Input: part model. Units: mm. Frame: model coordinates. A direction names the side the tool comes from. Round coordinates to 2 decimals unless told otherwise and drop trailing zeros. Loops run counter-clockwise (first coordinate to the right, second up) from the corner with the lowest first, then second, coordinate; pieces in that order, holes last. Notation, with made-up numbers: M 49.25,-27.75 L 83.25,-27.75 A21 cw 83.25,-19.75 Z; hole C 29.25,53 d4. An arc over 180 degrees is marked long. Use one line per item in the form item = value. Start each with the question number.
Q1. Access query for faces 1 (the cylindrical face through (-46.122, -24.331, -26.533)), 2 (the cylindrical face through (55.506, 7.509, -23.846)), 3 (the flat face through (73.5, -8, -24)), 4 (the flat face through (-19, 22, 6)), 5 (the flat face through (-73.5, -15, -15)). Directions: +Z, -Z, +X, -X, +Y, -Y. A direction counts if a zero-diameter tool reaches every point of the face in a straight line with its end or side. Return the directions, or none.
Q2. First-contact query: P1, Ø24.5, axis at y = 6, z = -4, coming from the +X side; P2, Ø3.5, axis at x = -6, y = 22.5, coming from the -Z side; P3, Ø8, axis at x = -39.5, y = 9, coming from the +Z side; P4, Ø3.5, axis at x = 2.5, z = 2.5, coming from the -Y side. Flat tips, straight axial feed; report the tip coordinate or a pass-through.
Q3. Section query A-A, the plane z = 0. Output: boundary loops of the cut face in (x, y).
Q4. Section query C-C, the plane x = -5. Output: boundary loops of the cut face in (y, z), and give its area (3 significant figures).
Q5. Section query B-B, the plane y = 0. Output: boundary loops of the cut face in (x, z), and give its area (3 significant figures).
Q6. Mould query, pull axis Y, two halves, no side actions, for faces 6 (the cylindrical face through (27.65, 37.18, 4.88)), 7 (the flat face through (-19.5, -14, 34)), 8 (the cylindrical face through (-17.73, -20.983, 0.838)). Classes: pulls with the +Y half, pulls with the -Y half, needs draft (parallel to the pull), parting line crosses it, or undercut.
Q7. Section query D-D, the plane y = 32. Output: boundary loops of the cut face in (x, z), and give its area (3 significant figures).
Q8. Ray query, line 1 along Z through (x, y) = (51.5, 0); line 2 along Z through (x, y) = (14, 4). Return the intervals inside material, ascending.
```python
from build123d import *

# Parameters (mm, degrees)
SKETCH1_R           = 37.5
BOSS_EXTRUDE1_DEPTH = 73.5
SKETCH2_R           = 21
CUT_EXTRUDE1_DEPTH  = 157.273798188
SKETCH3_R           = 25
CUT_EXTRUDE2_DEPTH  = 36.5
SKETCH4_W           = 12
SKETCH4_H           = 20.96554604
CUT_EXTRUDE3_DEPTH  = 110.5
FILLET1_R           = 0.5
SKETCH5_W           = 54
SKETCH5_H           = 1.5


with BuildPart() as part:
    # Sketch1 → Boss-Extrude1 (new, symmetric)
    with BuildSketch(Plane(origin=(0, 0, 0), x_dir=(0, 0, -1), z_dir=(1, 0, 0))):
        Circle(SKETCH1_R)
    extrude(amount=BOSS_EXTRUDE1_DEPTH, both=True)

    # Sketch2 → Cut-Extrude1 (cut, through all)
    with BuildSketch(Plane(origin=(73.5, 0, 0), x_dir=(0, 0, -1), z_dir=(1, 0, 0))):
        Circle(SKETCH2_R)
    extrude(amount=-CUT_EXTRUDE1_DEPTH, mode=Mode.SUBTRACT)

    # Sketch3 → Cut-Extrude2 (cut)
    with BuildSketch(Plane(origin=(73.5, 0, 0), x_dir=(0, 0, -1), z_dir=(1, 0, 0))):
        Circle(SKETCH3_R)
    extrude(amount=-CUT_EXTRUDE2_DEPTH, mode=Mode.SUBTRACT)

    # Sketch4 → Cut-Extrude3 (cut)
    with BuildSketch(Plane.ZY.offset(73.5)):
        with Locations((0, 13.81722698)):
            Rectangle(SKETCH4_W, SKETCH4_H)
    extrude(amount=-CUT_EXTRUDE3_DEPTH, mode=Mode.SUBTRACT)

    # Fillet1
    fillet1_edges = [part.edges().sort_by_distance(p)[0] for p in [
        (37, -21, 0),
    ]]
    fillet(fillet1_edges, radius=FILLET1_R)

    # Sketch5 → Cut-Revolve1 (revolve, cut)
    with BuildSketch(Plane.XY, mode=Mode.PRIVATE) as cut_revolve1_sk:
        with Locations((-46.5, 36.75)):
            Rectangle(SKETCH5_W, SKETCH5_H)
    revolve(cut_revolve1_sk.sketch.rotate(Axis((-73.5, 0, 0), (1, 0, 0)), 90), axis=Axis((-73.5, 0, 0), (1, 0, 0)), mode=Mode.SUBTRACT)


solid = part.part
```
Results found:
q1.face_1 = -X
q1.face_2 = +X
q1.face_3 = +Z, -Z, +X, +Y, -Y
q1.face_4 = +X, -X
q1.face_5 = +Z, -Z, -X, +Y, -Y
q2.P1 = through
q2.P2 = -31.24
q2.P3 = 35.65
q2.P4 = -37.49
q3.outline = M -73.5,-36 L -19.5,-36 L -19.5,-37.5 L 73.5,-37.5 L 73.5,-25 L 37,-25 L 37,-21.5 A0.5 ccw 36.5,-21 L -73.5,-21 Z; M -73.5,24.3 L 37,24.3 L 37,25 L 73.5,25 L 73.5,37.5 L -19.5,37.5 L -19.5,36 L -73.5,36 Z
q4.outline = C 0,0 d75; hole M 20.12,-6 L 24.3,-6 L 24.3,6 L 20.12,6 A21 ccw long Z
q4.area = 2,990 mm²
q5.outline = M -73.5,-36 L -19.5,-36 L -19.5,-37.5 L 73.5,-37.5 L 73.5,-25 L 37,-25 L 37,-21.5 A0.5 ccw 36.5,-21 L -73.5,-21 Z; M -73.5,21 L 36.5,21 A0.5 ccw 37,21.5 L 37,25 L 73.5,25 L 73.5,37.5 L -19.5,37.5 L -19.5,36 L -73.5,36 Z
q5.area = 4,400 mm²
q6.face_6 = parting line crosses it
q6.face_7 = needs draft
q6.face_8 = undercut
q7.outline = M -73.5,-16.49 L -19.5,-16.49 L -19.5,-19.55 L 73.5,-19.55 L 73.5,19.55 L -19.5,19.55 L -19.5,16.49 L -73.5,16.49 Z
q7.area = 5,420 mm²
q8.line_1 = -37.5 to -25, 25 to 37.5
q8.line_2 = -37.29 to -20.62, 20.62 to 37.29
